```python
from build123d import *

# Parameters (mm, degrees)
SKETCH1_W            = 630
SKETCH1_H            = 579
BOSS_EXTRUDE1_DEPTH  = 1.5
CUT_EXTRUDE1_DEPTH   = 428.836709505
SKETCH3_W            = 30.414213562
SKETCH3_H            = 60
CUT_EXTRUDE2_DEPTH   = 428.836709505
M5_CLEARANCE_HOLE1_D = 5.8


with BuildPart() as part:
    # Sketch1 → Boss-Extrude1 (new, symmetric)
    with BuildSketch(Plane(origin=(0, 0, 0), x_dir=(0, 0, -1), z_dir=(1, 0, 0))):
        Rectangle(SKETCH1_W, SKETCH1_H)
    extrude(amount=BOSS_EXTRUDE1_DEPTH, both=True)

    # Sketch2 → Cut-Extrude1 (cut, through all)
    with BuildSketch(Plane.ZY.offset(1.5)):
        Polygon((-224, 289.5), (-224, 259.085786438), (-284.585786438, 198.5), (-315, 198.5), (-315, 289.5), align=None)
        Polygon((224, 289.5), (224, 259.085786438), (284.585786438, 198.5), (315, 198.5), (315, 289.5), align=None)
    extrude(amount=-CUT_EXTRUDE1_DEPTH, mode=Mode.SUBTRACT)

    # Sketch3 → Cut-Extrude2 (cut, through all)
    with BuildSketch(Plane.ZY.offset(1.5)):
        with Locations((299.792893219, 168.5)):
            Rectangle(SKETCH3_W, SKETCH3_H)
        with Locations((299.792893219, -199.5)):
            Rectangle(SKETCH3_W, SKETCH3_H)
    extrude(amount=-CUT_EXTRUDE2_DEPTH, mode=Mode.SUBTRACT)

    # M5 Clearance Hole1 (through all)
    with Locations(Plane.ZY.offset(1.5)):
        with Locations((-164, 274.5), (0, 274.5), (164, 274.5), (300, 78.5), (300, -109.5), (300, -259.5), (-300, -229.5), (-300, -45.5), (-300, 138.5)):
            Hole(M5_CLEARANCE_HOLE1_D / 2)


solid = part.part
```
Read the model definition and answer for the solid it produces. Units are mm, in the model's axes. Coordinates: 2 decimals unless noted, no trailing zeros. Answer as a JSON object with one key per item and string values.
Q1. Flat-ended cylindrical pins translate along their axes: pin 1 Ø1.5 at (x, y) = (0, 269.5) entering from -Z; pin 2 Ø1.5 at (x, z) = (0, -295.5) entering from +Y; pin 3 Ø5 at (y, z) = (-109.5, 300) entering from -X; pin 4 Ø1.5 at (x, z) = (0.5, 302) entering from +Y. Find the tip coordinate at first contact, or state that the pin passes through.
The answers:
{"pin 1": "stops at z = -224", "pin 2": "stops at y = 198.5", "pin 3": "passes through", "pin 4": "stops at y = 138.5"}
Q2. Determine the mould class of faces 1 (the flat face through (1.5, 4, 4)), 2 (the flat face through (-0.021, 229.217, -253.869)), 3 (the flat face through (-1.5, 4, 4)) for opening direction X: pulls with the +X half, pulls with the -X half, needs draft (parallel to the pull), parting line crosses it, or undercut.
The answers:
{"face 1": "pulls with the +X half", "face 2": "needs draft", "face 3": "pulls with the -X half"}
Q3. Consider line 1 (Z direction, x = 0.2, y = 274.5); line 2 (Y direction, x = -0.65, z = -300); line 3 (Y direction, x = 0.4, z = 300). Determine where each line is inside the solid, lowest interval first. Write a range as [from, to].
The answers:
{"line 1": "z = [-224, -166.9], [-161.1, -2.9], [2.9, 161.1], [166.9, 224]", "line 2": "y = [-289.5, -232.4], [-226.6, -48.4], [-42.6, 135.6], [141.4, 198.5]", "line 3": "y = [-289.5, -262.4], [-256.6, -229.5], [-169.5, -112.4], [-106.6, 75.6], [81.4, 138.5]"}
Q4. The part is cut by section A-A on x = -0.6. Give the number of separate pieces and of enclosed holes in the cut face, then the cut area to 3 significant figures.
The answers:
{"separate pieces": "1", "enclosed holes": "9", "area": "348,000 mm2"}
